Read the model definition and answer for the solid it produces. Units are mm, in the model's axes. A direction names the side the tool comes from. Coordinates: 2 decimals unless noted, no trailing zeros. Write each loop counter-clockwise with the first axis right and the second up, starting at its lowest first coordinate (ties: lowest second). Pieces come first, ordered by that corner, then holes. Notation, with made-up numbers: (-8.75, 30) -> (50.25, 30) arc R16 ccw to (50.25, 58) -> close; hole circle Ø4 at (-25, 55.5). An arc over 180 degrees is marked (long way). Answer as a JSON object with one key per item and string values. Group by question number.
(1) Straight lines are drawn through the part: L1, parallel to X at y = 0, z = 3.6; L2, parallel to Y at x = 0, z = 1.4; L3, parallel to X at y = -2.5, z = 2.15. For each, find the intervals that lie inside material, in ascending order.
(2) For a pull along Y with two mould halves and no side action, classify faces 1 (the face through (0, -6, 0)), 2 (the face through (58, 14, 2)), 3 (the face through (-25.18, -12.08, 2.46)) as +Y half, -Y half, draft (parallel to the pull), parting line (faces both ways), or undercut.
(3) Find section B-B (y = 0). Give the vertices of the cut face in (x, z), then the cut area to 3 significant figures.
(4) Find section D-D (z = 2.5). Count the separate pieces of the cut face and the enclosed holes in it, then the cut area to 3 significant figures.
(5) Find section C-C (x = -24). Give the vertices of the cut face in (y, z), then the cut area to 3 significant figures.
(6) Flat-ended cylindrical pins translate along their axes: P1, Ø2.5, axis at x = 0, y = 10, coming from the +Z side; P2, Ø2.5, axis at y = 13.5, z = 3.5, coming from the +X side. Find the tip coordinate at first contact, or state that the pin passes through.
(7) Which of the six approach directions +Z, -Z, +X, -X, +Y, -Y give full straight-line access (tool end or side, diameter ignored) to faces 4 (the face through (52.526, -0.481, 2.465)), 5 (the face through (-48, 12, 2))?
(8) Find section A-A (x = 20). Give the vertices of the cut face in (y, z), then the cut area to 3 significant figures.
Autodesk Inventor part; units mm, degrees
ref_plane "YZ Plane" through (0, 0, 0) normal (1, 0, 0) x (0, 1, 0)
ref_plane "XZ Plane" through (0, 0, 0) normal (0, 1, 0) x (-1, 0, 0)
ref_plane "XY Plane" through (0, 0, 0) normal (0, 0, 1) x (1, 0, 0)
sketch "Náčrt1" plane through (0, 0, 0) normal (0, 0, 1) x (1, 0, 0)
  line L0 (0, -21) -> (0, 21)
  line L1 (-82.8, 0) -> (83.8, 0)
  line L2 (57, -15) -> (-58, -15)
  line L3 (-59, -14) -> (-59, 14)
  line L4 (-58, 15) -> (57, 15)
  line L5 (60, 12) -> (60, -12)
  circle A0 centre (20, 0) radius 5
  circle A1 centre (-20, 0) radius 5
  circle A2 centre (-55.625, -11.625) radius 2.5
  circle A3 centre (-32.375, 11.625) radius 2.5
  circle A4 centre (-24, -11) radius 1.6
  circle A5 centre (0, 10) radius 1.6
  circle A6 centre (51, 0) radius 1.6
  circle A7 centre (31, -11) radius 1.6
  line L6 (6, -6) -> (6, 0)
  line L7 (1, 0) -> (1, -6)
  line L8 (-3.5, -6) -> (-3.5, 0)
  line L9 (-8.5, 0) -> (-8.5, -6)
  arc A8 (1, -6) -> (6, -6) centre (3.5, -6) ccw
  arc A9 (-8.5, -6) -> (-3.5, -6) centre (-6, -6) ccw
  line L10 (-58, -15) -> (-59, -14)
  line L11 (-59, 14) -> (-58, 15)
  line L12 (57, -15) -> (60, -12)
  line L13 (57, 15) -> (60, 12)
  circle A10 centre (0, 0) radius 5
  arc A11 (6, 0) -> (4.4286, 2.3212) centre (3.5, 0) ccw
  arc A12 (1, -4.899) -> (4.4286, 2.3212) centre (0, 0) ccw
  arc A13 (-4.5625, 2.0454) -> (-8.5, 0) centre (-6, 0) ccw
  arc A14 (4.4286, 2.3212) -> (-4.5625, 2.0454) centre (0, 0) ccw
  arc A15 (-3.5, -3.5707) -> (1, -4.899) centre (0, 0) ccw
  arc A16 (-4.5625, 2.0454) -> (-3.5, -3.5707) centre (0, 0) ccw
  arc A17 (1, -4.899) -> (4.4286, 2.3212) centre (0, 0) ccw
  line L14 (1, -4.899) -> (1, -6)
  line L15 (-3.5, -3.5707) -> (-3.5, -6)
  arc A18 (-3.5, 0) -> (-4.5625, 2.0454) centre (-6, 0) ccw
  arc A19 (4.4286, 2.3212) -> (1, 0) centre (3.5, 0) ccw
  line L16 (-48, 15) -> (-48, 9)
  line L17 (-40, 15) -> (-40, 9)
  arc A20 (-48, 9) -> (-40, 9) centre (-44, 9) ccw
  line L18 (-48, 15) -> (-40, 15)
  point P0 (60, -15)
  point P1 (-59, 15)
  point P2 (-59, -15)
  point P3 (60, 15)
  dimension "d0" = 30
  dimension "d1" = 119
  dimension "d2" = 10
  dimension "d3" = 40
  dimension "d5" = 5
  dimension "d6" = 3.375
  dimension "d7" = 3.375
  dimension "d8" = 3.375
  dimension "d9" = 26.625
  dimension "d10" = 40
  dimension "d11" = 35
  dimension "d12" = 4
  dimension "d13" = 3.2
  dimension "d14" = 59
  dimension "d15" = 5
  dimension "d16" = 9
  dimension "d17" = 29
  dimension "d18" = 5
  dimension "d19" = 4.5
  dimension "d21" = 50.5
  dimension "d22" = 6.5
  dimension "d23" = 1
  dimension "d24" = 1
  dimension "d25" = 1
  dimension "d26" = 1
  dimension "d27" = 3
  dimension "d28" = 3
  dimension "d29" = 3
  dimension "d30" = 3
  dimension "d33" = 10
  dimension "d34" = 8
  dimension "d35" = 10
  dimension "d36" = 15
extrude "Vysunutí1" add sketch "Náčrt1" along normal blind 5 contours L2 L10 L3 L1 A1 L9 A9 L8 A10 L0 | L0 A10 L7 A8 L6 L1 A0 A6 L5 L12 L2 | L8 A9 L9 L1 A10 | A10 L1 L6 A8 L7 | A10 A13 L1 A1 L3 L11 L4 L16 A20 L17 L0 A5 | L0 A5 L4 L13 L5 L1 A6 A0 A11 A10 | L1 A13 A10 | A10 A11 L1
equation "\"d7\" = d6"
equation "\"d8\" = d6"
Results below:
{
 "1": {"L1": "x = -59 to -25, -15 to -5, 5 to 15, 25 to 49.4, 52.6 to 60", "L2": "y = -15 to -5, 5 to 8.4, 11.6 to 15", "L3": "x = -59 to -24.33, -15.67 to -4.33, 4.33 to 15.67, 24.33 to 60"},
 "2": {"face 1": "draft", "face 2": "+Y half", "face 3": "undercut"},
 "3": {"outline": "(-59, 0) -> (-25, 0) -> (-25, 5) -> (-59, 5) -> close; (-15, 0) -> (-5, 0) -> (-5, 5) -> (-15, 5) -> close; (5, 0) -> (15, 0) -> (15, 5) -> (5, 5) -> close; (25, 0) -> (49.4, 0) -> (49.4, 5) -> (25, 5) -> close; (52.6, 0) -> (60, 0) -> (60, 5) -> (52.6, 5) -> close", "area": "429 mm2"},
 "4": {"separate pieces": "1", "enclosed holes": "9", "area": "3,180 mm2"},
 "5": {"outline": "(-15, 0) -> (-12.6, 0) -> (-12.6, 5) -> (-15, 5) -> close; (-9.4, 0) -> (-3, 0) -> (-3, 5) -> (-9.4, 5) -> close; (3, 0) -> (15, 0) -> (15, 5) -> (3, 5) -> close", "area": "104 mm2"},
 "6": {"P1": "passes through", "P2": "stops at x = 59.75"},
 "7": {"face 4": "+Z, -Z", "face 5": "+Z, -Z, +Y"},
 "8": {"outline": "(-15, 0) -> (-5, 0) -> (-5, 5) -> (-15, 5) -> close; (5, 0) -> (15, 0) -> (15, 5) -> (5, 5) -> close", "area": "100 mm2"}
}
